Here's how the part is built. I have some questions about the finished solid (model axes, mm). A direction names the side the tool comes from. Give positions to 0.01 mm unless a question says otherwise; leave off trailing zeros. Write each loop counter-clockwise with the first axis right and the second up, starting at its lowest first coordinate (ties: lowest second). Pieces come first, ordered by that corner, then holes. Notation, with made-up numbers: (-26.5, -4.75) - (-13.5, -4.75) arc R30 cw to (-13.5, 27.25) - close; hole circle Ø1 at (-19.5, 87). An arc over 180 degrees is marked (long way). Use a Markdown table: item, result.
```python
from build123d import *

# Parameters (mm, degrees)
SKETCH_W        = 120
SKETCH_H        = 35
PAD_DEPTH       = 5
POCKET_DEPTH    = 5
POCKET001_DEPTH = 5


with BuildPart() as part:
    # Sketch → Pad (new body)
    with BuildSketch(Plane.XY):
        Rectangle(SKETCH_W, SKETCH_H)
    extrude(amount=PAD_DEPTH)

    # Sketch001 (on Face6 of Pad) → Pocket (cut)
    with BuildSketch(Plane.XY.offset(5)):
        Polygon((40, -6.1), (60, -6.1), (60, 6.1), (40, 6.1), (36.445622, 0), align=None)
    extrude(amount=-POCKET_DEPTH, mode=Mode.SUBTRACT)

    # Sketch002 (on Face5 of Pocket) → Pocket001 (cut)
    with BuildSketch(Plane.XY.offset(5)):
        Polygon((20, 17.5), (10, 7.5), (-40, 7.5), (-60, -17.5), (-60, 17.5), align=None)
        Polygon((60, 17.5), (60, 12.5), (55, 17.5), align=None)
        Polygon((60, -17.5), (60, -12.5), (55, -17.5), align=None)
    extrude(amount=-POCKET001_DEPTH, mode=Mode.SUBTRACT)


solid = part.part
```
Item 1: Will this pin go through, and if not, where does the flat tip stop? pin 1 Ø3 at (x, z) = (-30.5, 3) entering from +Y.
Values:
| item | result |
|---|---|
| pin 1 | stops at y = 7.5 |
Item 2: If we section it at D-D, the plane x = -18.5: Write out the boundary of the cut face in (y, z).
Values:
| item | result |
|---|---|
| outline | (-17.5, 0) - (7.5, 0) - (7.5, 5) - (-17.5, 5) - close |
Item 3: If we section it at C-C, the plane y = -8: Write out the boundary of the cut face in (x, z), plus the area to 3 significant figures.
Values:
| item | result |
|---|---|
| outline | (-52.4, 0) - (60, 0) - (60, 5) - (-52.4, 5) - close |
| area | 562 mm2 |
Item 4: For faces 5 (the flat face through (60, 9, 2)), 6 (the flat face through (-15, 7.5, 3)), 7 (the flat face through (38.248, 3.093, 2.535)), which set-ups out of +Z, -Z, +X, -X, +Y, -Y let a thin tool reach every point of the face, with its end or its side?
Values:
| item | result |
|---|---|
| face 5 | +Z, -Z, +X, +Y, -Y |
| face 6 | +Z, -Z, -X, +Y |
| face 7 | +Z, -Z, +X |
Item 5: If we section it at B-B, the plane z = 4: Write out the boundary of the cut face in (x, y), plus the area to 3 significant figures.
Values:
| item | result |
|---|---|
| outline | (-60, -17.5) - (55, -17.5) - (60, -12.5) - (60, -6.1) - (40, -6.1) - (36.45, 0) - (40, 6.1) - (60, 6.1) - (60, 12.5) - (55, 17.5) - (20, 17.5) - (10, 7.5) - (-40, 7.5) - close |
| area | 2,910 mm2 |
Item 6: Thinking about a two-plate mould opening in Y: for faces 1 (the flat face through (38.2, -3.01, 2.54)), 2 (the flat face through (-1, -4, 0)), 3 (the flat face through (15.1, 12.6, 2.5)), 4 (the flat face through (50, -6.1, 3)), which applies, +Y half, -Y half, draft (parallel to the pull), parting line (faces both ways), or undercut?
Values:
| item | result |
|---|---|
| face 1 | undercut |
| face 2 | draft |
| face 3 | +Y half |
| face 4 | undercut |
Item 7: I need wall thicknesses on line 1 along Y through (x, z) = (54, 2.8); line 2 along Y through (x, z) = (-20.5, 3.9); line 3 along X through (y, z) = (3, 2.3). Which ranges of each line are inside material? Lowest first, please. Write a range as [from, to].
Values:
| item | result |
|---|---|
| line 1 | y = [-17.5, -6.1], [6.1, 17.5] |
| line 2 | y = [-17.5, 7.5] |
| line 3 | x = [-43.6, 38.19] |
Item 8: If we section it at A-A, the plane x = 45: Write out the boundary of the cut face in (y, z).
Values:
| item | result |
|---|---|
| outline | (-17.5, 0) - (-6.1, 0) - (-6.1, 5) - (-17.5, 5) - close; (6.1, 0) - (17.5, 0) - (17.5, 5) - (6.1, 5) - close |
